Could you check a few things on this model? Use its own coordinates, in mm. A direction names the side the tool comes from. Give positions to 0.01 mm unless a question says otherwise; leave off trailing zeros. Write each loop counter-clockwise with the first axis right and the second up, starting at its lowest first coordinate (ties: lowest second). Pieces come first, ordered by that corner, then holes. Notation, with made-up numbers: M 70.5,-38 L 104.5,-38 A19 ccw 104.5,-8 Z; hole C 72,45 d9. An arc over 180 degrees is marked long. Use one line per item in the form item = value.
from build123d import *

# Parameters (mm, degrees)
F0_W        = 254
F0_H        = 254
F0_R        = 25.4
F1_DEPTH    = 220.472
F2_DEPTH    = 144.272
F3_R        = 25.4
F4_DEPTH    = 135.89
F5_W        = 241.9015839696
F5_H        = 233.4794849157
F5_W_2      = 228.9127036929
F5_H_2      = 217.6413685083
F6_DEPTH    = 101.6
F6_FACE_W   = 241.9015839696
F6_FACE_H   = 233.4794849157
F6_FACE_W_2 = 228.9127036929
F6_FACE_H_2 = 217.6413685083
F7_DEPTH    = 25.4
F8_W        = 228.178890729
F8_H        = 17.78
F8_W_2      = 17.693109271
F9_DEPTH    = 76.2
F8_H_2      = 218.44
F10_DEPTH   = 296.672


with BuildPart() as f1:
    # F0 (on Right) → F1 (new body)
    with BuildSketch(Plane.YZ):
        with Locations((0, 15.5562520722)):
            Rectangle(F0_W, F0_H)
        Circle(F0_R, mode=Mode.SUBTRACT)
        Circle(F0_R)
    extrude(amount=F1_DEPTH)

    # F0 (on Right) → F2 (cut)
    with BuildSketch(Plane.YZ):
        Circle(F0_R)
    extrude(amount=F2_DEPTH, mode=Mode.SUBTRACT)

    # F3 (on face) → F4 (cut)
    with BuildSketch(Plane.XY.offset(142.5562520722)):
        with Locations((101.4855039687, 0)):
            Circle(F3_R)
    extrude(amount=-F4_DEPTH, mode=Mode.SUBTRACT)

    # F5 (on face) → F6 (join)
    with BuildSketch(Plane.YZ):
        with Locations((0.4678927362, 20.2352032065)):
            Rectangle(F5_W, F5_H)
        with Locations((0.4346482456, 20.9778919816)):
            Rectangle(F5_W_2, F5_H_2, mode=Mode.SUBTRACT)
    extrude(amount=-F6_DEPTH)

    # F6_face (on face) + F0 (on Right) → F7 (join)
    with BuildSketch(Plane(origin=(-101.6, 0.7166497245, 14.6779207971), x_dir=(0, 1, 0), z_dir=(-1, 0, 0))):
        with Locations((-0.2487569883, -5.5572824094)):
            Rectangle(F6_FACE_W, F6_FACE_H)
        with Locations((-0.282001479, -6.2999711845)):
            Rectangle(F6_FACE_W_2, F6_FACE_H_2, mode=Mode.SUBTRACT)
    with BuildSketch(Plane.YZ):
        with Locations((0, 15.5562520722)):
            Rectangle(F0_W, F0_H)
        Circle(F0_R, mode=Mode.SUBTRACT)
    extrude(amount=F7_DEPTH, dir=(-1, 0, 0))

    # F8 (on face) → F9 (join)
    with BuildSketch(Plane.XY.offset(142.5562520722)):
        with Locations((88.6894453645, 118.11)):
            Rectangle(F8_W, F8_H)
        with Locations((211.6254453645, 118.11)):
            Rectangle(F8_W_2, F8_H)
        with Locations((88.6894453645, -118.11)):
            Rectangle(F8_W, F8_H)
        with Locations((211.6254453645, -118.11)):
            Rectangle(F8_W_2, F8_H)
    extrude(amount=F9_DEPTH)

    # F8 (on face) → F10 (join)
    with BuildSketch(Plane.XY.offset(142.5562520722)):
        with Locations((211.6254453645, 0)):
            Rectangle(F8_W_2, F8_H_2)
    extrude(amount=F10_DEPTH)


solid = f1.part
1) If I drill on L1, parallel to Z at x = -33.5, y = 84; L2, parallel to X at y = 0, z = 87.5; L3, parallel to Z at x = 6.5, y = 2, over which ranges is the centre line in solid material (lowest first)?
Checked values:
L1 = -96.5 to -87.84, 129.8 to 136.97
L2 = -25.4 to 76.09, 126.89 to 220.47
L3 = -111.44 to -25.32, 25.32 to 142.56
2) I want a section at B-B, the plane y = 0. Please give me the cut outline in (x, z).
Checked values:
outline = M -127,-96.5 L -25.4,-96.5 L -25.4,-111.44 L 220.47,-111.44 L 220.47,439.23 L 202.78,439.23 L 202.78,142.56 L 126.89,142.56 L 126.89,25.4 L 144.27,25.4 L 144.27,-25.4 L -25.4,-25.4 L -25.4,-87.84 L -127,-87.84 Z; M -127,129.8 L -25.4,129.8 L -25.4,25.4 L 76.09,25.4 L 76.09,142.56 L -25.4,142.56 L -25.4,136.97 L -127,136.97 Z
3) I want a section at A-A, the plane x = 133.5. Please give me the cut outline in (y, z), plus the area to 3 significant figures.
Checked values:
outline = M -127,-111.44 L 127,-111.44 L 127,218.76 L 109.22,218.76 L 109.22,142.56 L -109.22,142.56 L -109.22,218.76 L -127,218.76 Z; hole C 0,0 d50.8
area = 65,200 mm2
4) Thinking about a two-plate mould opening in Z: for faces 1 (the flat face through (96, 118, 218.756)), 2 (the flat face through (-25.4, -1, 47)), 3 (the flat face through (212, -109.22, 327)), 4 (the flat face through (99, -2, -111.444)), which applies, released by +Z, released by -Z, zero draft, split by the parting line, or undercut?
Checked values:
face_1 = released by +Z
face_2 = undercut
face_3 = zero draft
face_4 = released by -Z
5) For faces 5 (the flat face through (87, 109.22, 180)), 6 (the flat face through (-75, -114.022, 23)), 7 (the flat face through (-75, -1, -96.505)), which set-ups out of +Z, -Z, +X, -X, +Y, -Y let a thin tool reach every point of the face, with its end or its side?
Checked values:
face_5 = +Z, -X
face_6 = -X
face_7 = -Z, -X, +Y, -Y
6) I want a section at D-D, the plane y = 58.5. Please give me the cut outline in (x, z), plus the area to 3 significant figures.
Checked values:
outline = M -127,-96.5 L -25.4,-96.5 L -25.4,-111.44 L 220.47,-111.44 L 220.47,439.23 L 202.78,439.23 L 202.78,142.56 L -25.4,142.56 L -25.4,136.97 L -127,136.97 L -127,129.8 L -25.4,129.8 L -25.4,-87.84 L -127,-87.84 Z
area = 69,300 mm2
7) For pin 1 Ø2 at (y, z) = (-53.5, 103) entering from -X; pin 2 Ø15 at (y, z) = (6, 2.5) entering from -X; pin 3 Ø14 at (x, y) = (50, 119.5) entering from +Z, each with a flat end and sliding along its axis, tell me the tip position at first contact or that it passes through.
Checked values:
pin_1 = -25.4
pin_2 = 144.27
pin_3 = 218.76
8) I want a section at C-C, the plane z = 82.5. Please give me the cut outline in (x, y), plus the area to 3 significant figures.
Checked values:
outline = M -127,-120.48 L -25.4,-120.48 L -25.4,-127 L 220.47,-127 L 220.47,127 L -25.4,127 L -25.4,121.42 L -127,121.42 L -127,114.89 L -25.4,114.89 L -25.4,-114.02 L -127,-114.02 Z; hole C 101.49,0 d50.8
area = 61,700 mm2
